from build123d import *

# Parameters (mm, degrees)
EXTRUDE_1_DEPTH     = 5
CUT_EXTRUDE_1_DEPTH = 5


with BuildPart() as part:
    # 草图1 → 凸台-拉伸1 (new body)
    with BuildSketch(Plane.XY):
        Polygon((145, 10), (0, 10), (-145, 10), (-145, -10), (145, -10), align=None)
    extrude(amount=EXTRUDE_1_DEPTH)

    # 草图3 → 切除-拉伸1 (cut)
    with BuildSketch(Plane(origin=(0, 0, 0), x_dir=(-1, 0, 0), z_dir=(0, 0, -1))):
        with BuildLine():
            Line((-135, 5), (-135, 0))
            Line((-135, 0), (-132.25, 0))
            Line((-132.25, 0), (-132.25, 5))
            ThreePointArc((-132.25, 5), (-133.055456352, 6.944543648), (-135, 7.75))
            Line((-135, 7.75), (-135, 5))
        make_face()
        with BuildLine():
            Line((-137.75, 5), (-137.75, 0))
            Line((-137.75, 0), (-135, 0))
            Line((-135, 0), (-135, 5))
            Line((-135, 5), (-135, 7.75))
            ThreePointArc((-135, 7.75), (-136.944543648, 6.944543648), (-137.75, 5))
        make_face()
        with BuildLine():
            Line((-135, 0), (-137.75, 0))
            Line((-137.75, 0), (-137.75, -5))
            ThreePointArc((-137.75, -5), (-136.944543648, -6.944543648), (-135, -7.75))
            Line((-135, -7.75), (-135, -5))
            Line((-135, -5), (-135, 0))
        make_face()
        with BuildLine():
            Line((-132.25, 0), (-135, 0))
            Line((-135, 0), (-135, -5))
            Line((-135, -5), (-135, -7.75))
            ThreePointArc((-135, -7.75), (-133.055456352, -6.944543648), (-132.25, -5))
            Line((-132.25, -5), (-132.25, 0))
        make_face()
        with BuildLine():
            Line((-125, 0), (-127.75, 0))
            ThreePointArc((-127.75, 0), (-126.944543648, -1.944543648), (-125, -2.75))
            Line((-125, -2.75), (125, -2.75))
            ThreePointArc((125, -2.75), (126.944543648, -1.944543648), (127.75, 0))
            Line((127.75, 0), (125, 0))
            Line((125, 0), (-125, 0))
        make_face()
        with BuildLine():
            ThreePointArc((-125, 2.75), (-126.944543648, 1.944543648), (-127.75, 0))
            Line((-127.75, 0), (-125, 0))
            Line((-125, 0), (125, 0))
            Line((125, 0), (127.75, 0))
            ThreePointArc((127.75, 0), (126.944543648, 1.944543648), (125, 2.75))
            Line((125, 2.75), (-125, 2.75))
        make_face()
        with BuildLine():
            Line((135, 5), (135, 0))
            Line((135, 0), (137.75, 0))
            Line((137.75, 0), (137.75, 5))
            ThreePointArc((137.75, 5), (136.944543648, 6.944543648), (135, 7.75))
            Line((135, 7.75), (135, 5))
        make_face()
        with BuildLine():
            Line((132.25, 5), (132.25, 0))
            Line((132.25, 0), (135, 0))
            Line((135, 0), (135, 5))
            Line((135, 5), (135, 7.75))
            ThreePointArc((135, 7.75), (133.055456352, 6.944543648), (132.25, 5))
        make_face()
        with BuildLine():
            Line((135, 0), (132.25, 0))
            Line((132.25, 0), (132.25, -5))
            ThreePointArc((132.25, -5), (133.055456352, -6.944543648), (135, -7.75))
            Line((135, -7.75), (135, -5))
            Line((135, -5), (135, 0))
        make_face()
        with BuildLine():
            Line((137.75, 0), (135, 0))
            Line((135, 0), (135, -5))
            Line((135, -5), (135, -7.75))
            ThreePointArc((135, -7.75), (136.944543648, -6.944543648), (137.75, -5))
            Line((137.75, -5), (137.75, 0))
        make_face()
    extrude(amount=-CUT_EXTRUDE_1_DEPTH, mode=Mode.SUBTRACT)


solid = part.part
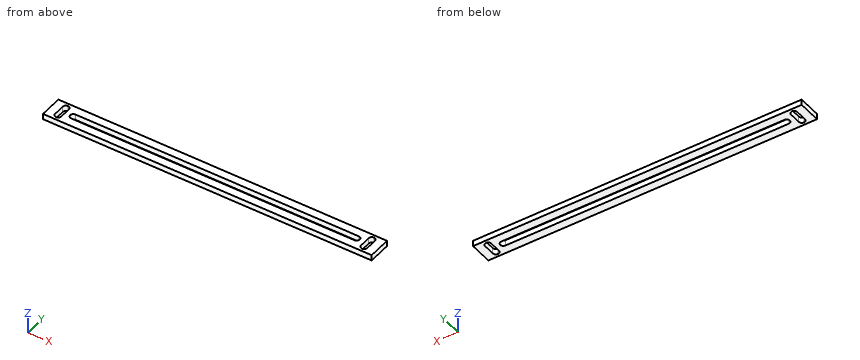
Can you work these out from the model? Positions are in its coordinate system, mm. Give positions to 0.01 mm unless a question says otherwise; leave off trailing zeros. Order: outer loops, then holes, each group sorted by start corner. A loop starts at its lowest first (then second) coordinate and runs counter-clockwise, first axis right, second up. Notation, with made-up numbers: M 16.5,34.25 L 33.5,34.25 A20 cw 33.5,60.25 Z; hole C -6.5,32 d11. An arc over 180 degrees is marked long. Use a Markdown table: item, result. Add a question column.
Item 1: If I drill on L1, parallel to X at y = 0.5, z = 3; L2, parallel to X at y = -3.25, z = 4.45; L3, parallel to Y at x = 36.5, z = 2.35, over which ranges is the centre line in solid material (lowest first)? Write a range as [from, to].
Item 2: Suppose I cut it at A-A (x = -114). List the corners of the cut face in (y, z) for me.
Item 3: Suppose I cut it at B-B (z = 0.9). List the corners of the cut face in (x, y) for me, then the cut area to 3 significant figures.
Answer sheet:
| question | item | result |
|---|---|---|
| 1 | L1 | x = [-145, -137.75], [-132.25, -127.7], [127.7, 132.25], [137.75, 145] |
| 1 | L2 | x = [-145, -137.75], [-132.25, 132.25], [137.75, 145] |
| 1 | L3 | y = [-10, -2.75], [2.75, 10] |
| 2 | outline | M -10,0 L -2.75,0 L -2.75,5 L -10,5 Z; M 2.75,0 L 10,0 L 10,5 L 2.75,5 Z |
| 3 | outline | M -145,-10 L 145,-10 L 145,10 L -145,10 Z; hole M -137.75,-5 A2.75 ccw -132.25,-5 L -132.25,5 A2.75 ccw -137.75,5 Z; hole M -125,-2.75 L 125,-2.75 A2.75 ccw 125,2.75 L -125,2.75 A2.75 ccw Z; hole M 132.25,-5 A2.75 ccw 137.75,-5 L 137.75,5 A2.75 ccw 132.25,5 Z |
| 3 | area | 4,240 mm² |
